Geometry check sheet. Reference: the model listing, model coordinates, mm. Coordinates: 2 decimals unless noted, no trailing zeros. Loops run counter-clockwise (first coordinate to the right, second up) from the corner with the lowest first, then second, coordinate; pieces in that order, holes last.
from build123d import *

# Parameters (mm, degrees)
F0_W     = 20
F0_H     = 328.5
F0_W_2   = 6.1
F0_H_2   = 12
F1_DEPTH = 5
F2_DEPTH = 8
F3_R     = 1


with BuildPart() as f1:
    # F0 (on Top) → F1 (new body)
    with BuildSketch(Plane.XY):
        Rectangle(F0_W, F0_H)
        Rectangle(F0_W_2, F0_H_2, mode=Mode.SUBTRACT)
    extrude(amount=F1_DEPTH)

    # F0 (on Top) → F2 (join)
    with BuildSketch(Plane.XY):
        Rectangle(F0_W_2, F0_H_2)
    extrude(amount=F2_DEPTH)

    # F3
    f3_edges = [f1.edges().sort_by_distance(p)[0] for p in [
        (3.05, 0, 8),
        (-3.05, 0, 8),
        (0, 6, 8),
        (0, -6, 8),
        (-10, 0, 0),
        (10, 0, 0),
        (-10, -164.25, 2.5),
        (10, -164.25, 2.5),
        (10, 164.25, 2.5),
        (-10, 164.25, 2.5),
    ]]
    fillet(f3_edges, radius=F3_R)


solid = f1.part
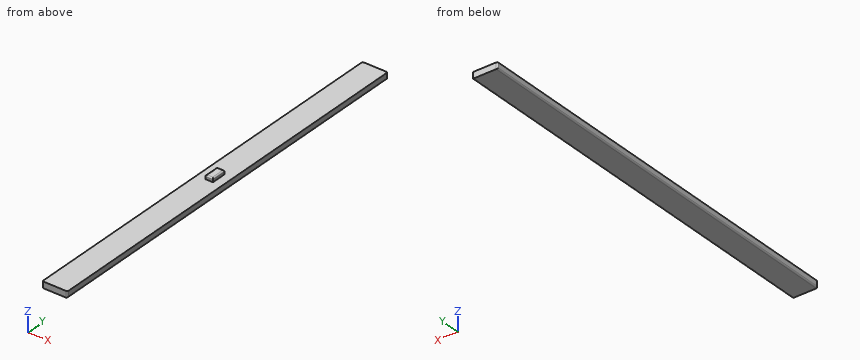
1) Depth check by flat-ended pin: pin 1 (5 mm diameter, centred on x = -7.5, y = 79.5, fed in from +Z); pin 2 (0.6 mm diameter, centred on x = -1, z = 6.5, fed in from +Y). Enter the tip coordinate at first touch or a pass-through.
Data:
pin 1: stops at z = 5
pin 2: stops at y = 6
2) Section check A-A on y = 88. Record the cut outline in (x, z).
Data:
outline: (-10, 1) arc R1 ccw to (-9, 0) - (9, 0) arc R1 ccw to (10, 1) - (10, 5) - (-10, 5) - close
3) Material ranges on probe 1 along Z at (x, y) = (5.25, -81); probe 2 along Y at (x, z) = (1.5, 6.25); probe 3 along Y at (x, z) = (1.75, 7.5), recorded low to high.
Data:
probe 1: z = 0 to 5
probe 2: y = -6 to 6
probe 3: y = -5.87 to 5.87
